Read the model definition and answer for the solid it produces. Units are mm, in the model's axes. Round coordinates to 2 decimals unless told otherwise and drop trailing zeros. Loops run counter-clockwise (first coordinate to the right, second up) from the corner with the lowest first, then second, coordinate; pieces in that order, holes last. Notation, with made-up numbers: M -13,88.5 L 27,88.5 A23 cw 27,117.5 Z; hole C 16.5,2 d7. An arc over 180 degrees is marked long. Write each question's results on one line, items separated by ' | '.
```python
from build123d import *

# Parameters (mm, degrees)
F0_R     = 11.0236
F1_DEPTH = 6.35


with BuildPart() as f1:
    # F0 (on Top) → F1 (new body)
    with BuildSketch(Plane.XY):
        with BuildLine():
            ThreePointArc((-37.058964, 0.270715), (-34.958103, -0.659612), (-32.713622, -1.150971))
            ThreePointArc((-32.713622, -1.150971), (-24.555801, 1.052314), (-20.140829, 8.257349))
            ThreePointArc((-20.140829, 8.257349), (-22.501454, 13.038914), (-23.340718, 18.304989))
            ThreePointArc((-23.340718, 18.304989), (-40.501055, 17.123743), (-37.058964, 0.270715))
        make_face()
        Polygon((-40.369035, 8.29814), (-37.53676, 17.014987), (-28.571611, 18.920588), (-22.438737, 12.109342), (-25.271013, 3.392495), (-34.236162, 1.486894), align=None, mode=Mode.SUBTRACT)
        with BuildLine():
            ThreePointArc((-14.881645, 3.285458), (-14.220455, 5.480534), (-13.237485, 7.551595))
            ThreePointArc((-13.237485, 7.551595), (-19.286416, 19.773486), (-11.203704, 30.756834))
            ThreePointArc((-11.203704, 30.756834), (-11.429976, 33.0433), (-11.194384, 35.328824))
            ThreePointArc((-11.194384, 35.328824), (-20.029351, 28.787423), (-23.340718, 18.304989))
            ThreePointArc((-23.340718, 18.304989), (-22.501454, 13.038914), (-20.140829, 8.257349))
            ThreePointArc((-20.140829, 8.257349), (-17.766451, 5.501443), (-14.881645, 3.285458))
        make_face()
        with BuildLine():
            ThreePointArc((-14.077064, -16.603405), (-10.722318, -15.19686), (-7.723338, -13.138023))
            ThreePointArc((-7.723338, -13.138023), (-9.60666, -11.830879), (-11.272602, -10.256025))
            ThreePointArc((-11.272602, -10.256025), (-24.765533, -12.232129), (-32.713622, -1.150971))
            ThreePointArc((-32.713622, -1.150971), (-34.958103, -0.659612), (-37.058964, 0.270715))
            ThreePointArc((-37.058964, 0.270715), (-33.567876, -10.153242), (-24.621757, -16.541789))
            ThreePointArc((-24.621757, -16.541789), (-19.341881, -15.283936), (-14.077064, -16.603405))
        make_face()
        with BuildLine():
            ThreePointArc((-11.709315, -35.161513), (-10.175319, -33.450963), (-9.014427, -31.468173))
            ThreePointArc((-9.014427, -31.468173), (-8.24061, -29.146714), (-7.978669, -26.713741))
            ThreePointArc((-7.978669, -26.713741), (-9.621301, -20.810155), (-14.077064, -16.603405))
            ThreePointArc((-14.077064, -16.603405), (-19.341881, -15.283936), (-24.621757, -16.541789))
            ThreePointArc((-24.621757, -16.541789), (-28.801161, -33.227265), (-11.709315, -35.161513))
        make_face()
        Polygon((-20.366718, -35.828967), (-27.781711, -30.44166), (-26.823662, -21.326433), (-18.45062, -17.598515), (-11.035627, -22.985823), (-11.993676, -32.101049), align=None, mode=Mode.SUBTRACT)
        with BuildLine():
            ThreePointArc((11.440725, -18.518818), (11.139694, -14.893619), (10.10836, -11.405203))
            ThreePointArc((10.10836, -11.405203), (8.283213, -12.792419), (6.270634, -13.890167))
            ThreePointArc((6.270634, -13.890167), (3.980475, -27.333357), (-9.014427, -31.468173))
            ThreePointArc((-9.014427, -31.468173), (-10.175319, -33.450963), (-11.709315, -35.161513))
            ThreePointArc((-11.709315, -35.161513), (-0.716737, -35.062472), (8.123635, -28.528377))
            ThreePointArc((8.123635, -28.528377), (8.558917, -23.118218), (11.440725, -18.518818))
        make_face()
        with BuildLine():
            ThreePointArc((29.822209, -22.001726), (28.669409, -20.01422), (27.1424, -18.297429))
            ThreePointArc((27.1424, -18.297429), (19.247526, -15.284877), (11.440725, -18.518818))
            ThreePointArc((11.440725, -18.518818), (8.558917, -23.118218), (8.123635, -28.528377))
            ThreePointArc((8.123635, -28.528377), (20.318877, -38.107442), (30.838669, -26.713741))
            ThreePointArc((30.838669, -26.713741), (30.581665, -24.30354), (29.822209, -22.001726))
        make_face()
        Polygon((27.781711, -30.44166), (20.366718, -35.828967), (11.993676, -32.101049), (11.035627, -22.985823), (18.45062, -17.598515), (26.823662, -21.326433), align=None, mode=Mode.SUBTRACT)
        with BuildLine():
            ThreePointArc((13.970648, 6.08922), (14.725967, 3.924729), (15.148067, 1.67143))
            ThreePointArc((15.148067, 1.67143), (27.225602, -4.660815), (27.1424, -18.297429))
            ThreePointArc((27.1424, -18.297429), (28.669409, -20.01422), (29.822209, -22.001726))
            ThreePointArc((29.822209, -22.001726), (33.124908, -11.516557), (29.64244, -1.089717))
            ThreePointArc((29.64244, -1.089717), (24.631583, 0.996092), (21.147821, 5.158146))
            ThreePointArc((21.147821, 5.158146), (17.607028, 5.992097), (13.970648, 6.08922))
        make_face()
        with BuildLine():
            ThreePointArc((25.789352, 20.15974), (20.484595, 13.582198), (21.147821, 5.158146))
            ThreePointArc((21.147821, 5.158146), (24.631583, 0.996092), (29.64244, -1.089717))
            ThreePointArc((29.64244, -1.089717), (38.83731, 1.521051), (42.833886, 10.203741))
            ThreePointArc((42.833886, 10.203741), (39.026349, 18.720957), (30.140454, 21.563699))
            ThreePointArc((30.140454, 21.563699), (27.893989, 21.081495), (25.789352, 20.15974))
        make_face()
        Polygon((37.53676, 17.014987), (40.369035, 8.29814), (34.236162, 1.486894), (25.271013, 3.392495), (22.438737, 12.109342), (28.571611, 18.920588), align=None, mode=Mode.SUBTRACT)
        with BuildLine():
            ThreePointArc((-1.474025, 15.168548), (0.817935, 15.218035), (3.091386, 14.923168))
            ThreePointArc((3.091386, 14.923168), (12.845872, 24.452815), (25.789352, 20.15974))
            ThreePointArc((25.789352, 20.15974), (27.893989, 21.081495), (30.140454, 21.563699))
            ThreePointArc((30.140454, 21.563699), (21.189057, 27.944848), (10.196401, 27.854894))
            ThreePointArc((10.196401, 27.854894), (6.664238, 23.733836), (1.629347, 21.706728))
            ThreePointArc((1.629347, 21.706728), (-0.257952, 18.596938), (-1.474025, 15.168548))
        make_face()
        with BuildLine():
            ThreePointArc((-11.203704, 30.756834), (-6.58735, 23.679137), (1.629347, 21.706728))
            ThreePointArc((1.629347, 21.706728), (6.664238, 23.733836), (10.196401, 27.854894))
            ThreePointArc((10.196401, 27.854894), (11.117323, 30.364812), (11.43, 33.02))
            ThreePointArc((11.43, 33.02), (1.160408, 44.390943), (-11.194384, 35.328824))
            ThreePointArc((-11.194384, 35.328824), (-11.429976, 33.0433), (-11.203704, 30.756834))
        make_face()
        Polygon((9.165436, 33.02), (4.582718, 25.0825), (-4.582718, 25.0825), (-9.165436, 33.02), (-4.582718, 40.9575), (4.582718, 40.9575), align=None, mode=Mode.SUBTRACT)
        with BuildLine():
            ThreePointArc((10.10836, -11.405203), (13.898004, -6.253247), (15.24, 0))
            ThreePointArc((15.24, 0), (15.216999, 0.836978), (15.148067, 1.67143))
            ThreePointArc((15.148067, 1.67143), (14.725967, 3.924729), (13.970648, 6.08922))
            ThreePointArc((13.970648, 6.08922), (9.60666, 11.830879), (3.091386, 14.923168))
            ThreePointArc((3.091386, 14.923168), (0.817935, 15.218035), (-1.474025, 15.168548))
            ThreePointArc((-1.474025, 15.168548), (-8.283213, 12.792419), (-13.237485, 7.551595))
            ThreePointArc((-13.237485, 7.551595), (-14.220455, 5.480534), (-14.881645, 3.285458))
            ThreePointArc((-14.881645, 3.285458), (-14.725967, -3.924729), (-11.272602, -10.256025))
            ThreePointArc((-11.272602, -10.256025), (-9.60666, -11.830879), (-7.723338, -13.138023))
            ThreePointArc((-7.723338, -13.138023), (-0.817935, -15.218035), (6.270634, -13.890167))
            ThreePointArc((6.270634, -13.890167), (8.283213, -12.792419), (10.10836, -11.405203))
        make_face()
        Circle(F0_R, mode=Mode.SUBTRACT)
    extrude(amount=F1_DEPTH)


solid = f1.part
```
1. Find section A-A, the plane x = 24. Give the vertices of the cut face in (y, z), then the cut area to 3 significant figures.
Completed:
outline: M -37.18,0 L -33.19,0 L -33.19,6.35 L -37.18,6.35 Z; M -20.07,0 L -16.25,0 L -16.25,6.35 L -20.07,6.35 Z; M -1.04,0 L 7.3,0 L 7.3,6.35 L -1.04,6.35 Z; M 13.84,0 L 18.91,0 L 18.91,6.35 L 13.84,6.35 Z; M 21.9,0 L 26.79,0 L 26.79,6.35 L 21.9,6.35 Z | area: 166 mm2
2. Find section B-B, the plane y = -7. Give the vertices of the cut face in (x, z).
Completed:
outline: M -35.43,0 L -30.83,0 L -30.83,6.35 L -35.43,6.35 Z; M -13.54,0 L -8.52,0 L -8.52,6.35 L -13.54,6.35 Z; M 8.52,0 L 13.54,0 L 13.54,6.35 L 8.52,6.35 Z; M 28.33,0 L 32.5,0 L 32.5,6.35 L 28.33,6.35 Z
3. Given P1, Ø8, axis at x = -12, y = 17.5, coming from the -Z side; P2, Ø1.9, axis at x = 2, z = 4, coming from the -Y side; P3, Ø2, axis at x = 3.5, z = 5, coming from the -Y side; P4, Ø1, axis at y = -16.5, z = 5.5, coming from the +X side, each flat-ended and moving along its own axis, determine where each tip first touches the part or whether it passes through.
Completed:
P1: passes through | P2: stops at y = -34.36 | P3: stops at y = -33.62 | P4: stops at x = 32.59
4. Find the intervals of material crossed by L1, parallel to X at y = -2.5, z = 3.75; L2, parallel to Y at x = -20, z = 3.75; L3, parallel to X at y = 4.5, z = 3.75, in increasing order.
Completed:
L1: x = -36.82 to -32.54, -15.03 to -10.74, 10.74 to 15.03, 25.6 to 30.58 | L2: y = -38.13 to -35.67, -18.29 to -13.27, 8.06 to 28.83 | L3: x = -41.31 to -36.95, -24.91 to -21.5, -16.61 to -10.06, 10.06 to 24.91, 36.95 to 41.31
5. Find section D-D, the plane z = 4.25. Count the separate pieces of the cut face and the enclosed holes in it, then the cut area to 3 significant figures.
Completed:
separate pieces: 1 | enclosed holes: 11 | area: 1,940 mm2
6. Determine the mould class of faces 1 (the face through (-25.548, 15.563, 3.131)), 2 (the face through (-14.75, -3.83, 3.13)) for opening direction X: released by +X, released by -X, zero draft, split by the parting line, or undercut.
Completed:
face 1: undercut | face 2: undercut
7. Find section C-C, the plane x = 0. Give the vertices of the cut face in (y, z), then the cut area to 3 significant figures.
Completed:
outline: M -34.81,0 L -30.43,0 L -30.43,6.35 L -34.81,6.35 Z; M -15.24,0 L -11.02,0 L -11.02,6.35 L -15.24,6.35 Z; M 11.02,0 L 19.12,0 L 19.12,6.35 L 11.02,6.35 Z; M 21.59,0 L 25.08,0 L 25.08,6.35 L 21.59,6.35 Z; M 40.96,0 L 44.45,0 L 44.45,6.35 L 40.96,6.35 Z | area: 150 mm2
